Geometry: final body of the model. Coordinates: model frame, mm. Face numbers are marked on the shaded views. A direction names the side the tool comes from. Round coordinates to 2 decimals unless told otherwise and drop trailing zeros. Order: outer loops, then holes, each group sorted by start corner. A loop starts at its lowest first (then second) coordinate and runs counter-clockwise, first axis right, second up. Notation, with made-up numbers: M 5.5,-9 L 29.5,-9 A25 cw 29.5,8 Z; hole C 44.25,-30 d1. An arc over 180 degrees is marked long. Return JSON: item names as keys, results as strings. Group by question number.
Q1. Mould query, pull axis X, two halves, no side actions, for the marked faces 1, 2 and 3. Classes: released by +X, released by -X, zero draft, split by the parting line, or undercut.
Q2. Cut plane C-C on y = 13.5. Output: boundary loops of the cut face in (x, z).
Q3. Ray query, probe 1 along Y at (x, z) = (13, -51.5); probe 2 along Y at (x, z) = (-32, -42); probe 3 along X at (y, z) = (58.5, 15). Return the intervals inside material, ascending.
Q4. Cut plane B-B on x = 9. Output: boundary loops of the cut face in (y, z).
Q5. Access query for the marked faces 4 and 5. Directions: +Z, -Z, +X, -X, +Y, -Y. A direction counts if a zero-diameter tool reaches every point of the face in a straight line with its end or side. Return the directions, or none.
Q6. Contact query for flat-ended pins moving along their axis: pin 1 (5 mm diameter, centred on y = 52, z = -12, fed in from -X); pin 2 (2 mm diameter, centred on x = -25.5, z = -38, fed in from +Y); pin 3 (6 mm diameter, centred on y = 32.5, z = -47.5, fed in from -X). Output: stop coordinate, or through.
Q7. Cut plane A-A on z = -7. Output: boundary loops of the cut face in (x, y) (3 decimals).
```python
from build123d import *

# Parameters (mm, degrees)
F1_DEPTH = 67.31
F2_DEPTH = 25.4


with BuildPart() as f1:
    # F0 (on Top) → F1 (new body)
    with BuildSketch(Plane.XY):
        with BuildLine():
            ThreePointArc((-6.1162381901, 23.7623695284), (-5.7969324328, 26.1592759352), (-5.6902200774, 28.5750012845))
            ThreePointArc((-5.6902200774, 28.5750012845), (-9.5823604521, 42.6503078125), (-20.1528966427, 52.7263573954))
            Line((-20.1528966427, 52.7263573954), (-20.1528966427, 23.7623695284))
            Line((-20.1528966427, 23.7623695284), (-6.1162381901, 23.7623695284))
        make_face()
        with BuildLine():
            ThreePointArc((-20.1528966427, 52.7263573954), (-9.5823604521, 42.6503078125), (-5.6902200774, 28.5750012845))
            ThreePointArc((-5.6902200774, 28.5750012845), (-5.7969324328, 26.1592759352), (-6.1162381901, 23.7623695284))
            Line((-6.1162381901, 23.7623695284), (31.5828956664, 23.7623695284))
            Line((31.5828956664, 23.7623695284), (31.5828956664, 65.5721053481))
            Line((31.5828956664, 65.5721053481), (-20.1528966427, 65.5721053481))
            Line((-20.1528966427, 65.5721053481), (-20.1528966427, 52.7263573954))
        make_face()
        with BuildLine():
            Line((-20.1528966427, 23.7623695284), (-20.1528966427, 52.7263573954))
            ThreePointArc((-20.1528966427, 52.7263573954), (-57.7408795784, 16.6270512491), (-6.1162381901, 23.7623695284))
            Line((-6.1162381901, 23.7623695284), (-20.1528966427, 23.7623695284))
        make_face()
    extrude(amount=-F1_DEPTH)

    # F0 (on Top) → F2 (join)
    with BuildSketch(Plane.XY):
        with BuildLine():
            ThreePointArc((-6.1162381901, 23.7623695284), (-5.7969324328, 26.1592759352), (-5.6902200774, 28.5750012845))
            ThreePointArc((-5.6902200774, 28.5750012845), (-9.5823604521, 42.6503078125), (-20.1528966427, 52.7263573954))
            Line((-20.1528966427, 52.7263573954), (-20.1528966427, 23.7623695284))
            Line((-20.1528966427, 23.7623695284), (-6.1162381901, 23.7623695284))
        make_face()
        with BuildLine():
            ThreePointArc((-20.1528966427, 52.7263573954), (-9.5823604521, 42.6503078125), (-5.6902200774, 28.5750012845))
            ThreePointArc((-5.6902200774, 28.5750012845), (-5.7969324328, 26.1592759352), (-6.1162381901, 23.7623695284))
            Line((-6.1162381901, 23.7623695284), (31.5828956664, 23.7623695284))
            Line((31.5828956664, 23.7623695284), (31.5828956664, 65.5721053481))
            Line((31.5828956664, 65.5721053481), (-20.1528966427, 65.5721053481))
            Line((-20.1528966427, 65.5721053481), (-20.1528966427, 52.7263573954))
        make_face()
        with BuildLine():
            Line((-20.1528966427, 23.7623695284), (-20.1528966427, 52.7263573954))
            ThreePointArc((-20.1528966427, 52.7263573954), (-57.7408795784, 16.6270512491), (-6.1162381901, 23.7623695284))
            Line((-6.1162381901, 23.7623695284), (-20.1528966427, 23.7623695284))
        make_face()
    extrude(amount=F2_DEPTH)


solid = f1.part
```
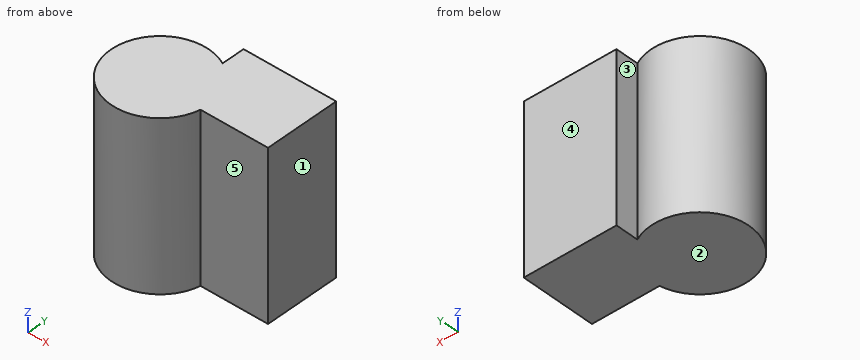
Result sheet:
{
 "1": {"face 1": "released by +X", "face 2": "zero draft", "face 3": "undercut"},
 "2": {"outline": "M -55.96,-67.31 L -10.21,-67.31 L -10.21,25.4 L -55.96,25.4 Z"},
 "3": {"probe 1": "y = 23.76 to 65.57", "probe 2": "y = 1.2 to 55.95", "probe 3": "x = -20.15 to 31.58"},
 "4": {"outline": "M 23.76,-67.31 L 65.57,-67.31 L 65.57,25.4 L 23.76,25.4 Z"},
 "5": {"face 4": "+Z, -Z, +X, -X, +Y", "face 5": "+Z, -Z, +X, -Y"},
 "6": {"pin 1": "stops at x = -50.77", "pin 2": "stops at y = 55.17", "pin 3": "stops at x = -60.47"},
 "7": {"outline": "M -20.153,52.726 A27.397 ccw long -6.116,23.762 L 31.583,23.762 L 31.583,65.572 L -20.153,65.572 Z"}
}
